from build123d import *

# Parameters (mm, degrees)
SKETCH1_W                 = 54.5
SKETCH1_H                 = 39
BOSS_EXTRUDE1_DEPTH       = 3
SKETCH10_R                = 7
CUT_EXTRUDE1_DEPTH        = 5
M2_CLEARANCE_HOLE1_D      = 2.4
M2_CLEARANCE_HOLE1_DEPTH  = 17
M2_CLEARANCE_HOLE1_TIP    = 0.721032743
SKETCH12_W                = 20
SKETCH12_H                = 5
BOSS_EXTRUDE2_DEPTH       = 20
SKETCH13_R                = 4.25
CUT_EXTRUDE2_DEPTH        = 5
SKETCH16_W                = 54.5
SKETCH16_H                = 5
BOSS_EXTRUDE4_DEPTH       = 12
F_8_CLEARANCE_HOLE1_D     = 4.4958
F_8_CLEARANCE_HOLE1_DEPTH = 17
F_8_CLEARANCE_HOLE1_TIP   = 1.350674586
RIB2_REACH                = 67.289
SKETCH20_WALL_W           = 150.605379482
SKETCH20_WALL_H           = 5
RIB4_REACH                = 67.289
SKETCH21_WALL_W           = 150.605379482
SKETCH21_WALL_H           = 5


with BuildPart() as part:
    # Sketch1 → Boss-Extrude1 (new body)
    with BuildSketch(Plane(origin=(0, 0, 0), x_dir=(1, 0, 0), z_dir=(0, 1, 0))):
        with Locations((-13.399543841, 8.129312584)):
            Rectangle(SKETCH1_W, SKETCH1_H)
    extrude(amount=BOSS_EXTRUDE1_DEPTH)

    # Sketch10 → Cut-Extrude1 (cut)
    with BuildSketch(Plane(origin=(0, 3, 0), x_dir=(1, 0, 0), z_dir=(0, 1, 0))):
        with Locations(Location((-13.399543841, 8.129312584, 0), (0, 0, 270))):
            Circle(SKETCH10_R)
    extrude(amount=-CUT_EXTRUDE1_DEPTH, mode=Mode.SUBTRACT)

    # M2 Clearance Hole1
    with Locations(Plane(origin=(-13.399543841, 3, -0.129312584), x_dir=(0, 0, 1), z_dir=(0, 1, 0))):
        with Locations((0, 0), (-8, 7.99475453), (-8, -7.99475453), (-16, 0)):
            Hole(M2_CLEARANCE_HOLE1_D / 2, depth=M2_CLEARANCE_HOLE1_DEPTH)
            with Locations((0, 0, -(M2_CLEARANCE_HOLE1_DEPTH + M2_CLEARANCE_HOLE1_TIP / 2))):  # 118° drill point
                Cone(0, M2_CLEARANCE_HOLE1_D / 2, M2_CLEARANCE_HOLE1_TIP, mode=Mode.SUBTRACT)

    # Sketch12 → Boss-Extrude2 (add)
    with BuildSketch(Plane(origin=(0, 3, 0), x_dir=(1, 0, 0), z_dir=(0, 1, 0))):
        with Locations((3.850456159, -8.870687416)):
            Rectangle(SKETCH12_W, SKETCH12_H)
        with Locations((-30.649543841, -8.870687416)):
            Rectangle(SKETCH12_W, SKETCH12_H)
    extrude(amount=BOSS_EXTRUDE2_DEPTH)

    # Sketch13 → Cut-Extrude2 (cut)
    with BuildSketch(Plane(origin=(0, 0, 6.370687416), x_dir=(-1, 0, 0), z_dir=(0, 0, -1))):
        with Locations((-3.850456159, 18)):
            Circle(SKETCH13_R)
        with Locations((30.649543841, 18)):
            Circle(SKETCH13_R)
    extrude(amount=-CUT_EXTRUDE2_DEPTH, mode=Mode.SUBTRACT)

    # Sketch16 → Boss-Extrude4 (add)
    with BuildSketch(Plane.XZ):
        with Locations((-13.399543841, 8.870687416)):
            Rectangle(SKETCH16_W, SKETCH16_H)
    extrude(amount=BOSS_EXTRUDE4_DEPTH)

    # #8 Clearance Hole1
    with Locations(Plane(origin=(-30.649543841, -8.2, 11.370687416), x_dir=(1, 0, 0), z_dir=(0, 0, 1))):
        with Locations((0, 0), (17.25, 0), (34.5, 0)):
            Hole(F_8_CLEARANCE_HOLE1_D / 2, depth=F_8_CLEARANCE_HOLE1_DEPTH)
            with Locations((0, 0, -(F_8_CLEARANCE_HOLE1_DEPTH + F_8_CLEARANCE_HOLE1_TIP / 2))):  # 118° drill point
                Cone(0, F_8_CLEARANCE_HOLE1_D / 2, F_8_CLEARANCE_HOLE1_TIP, mode=Mode.SUBTRACT)

    # Sketch20 wall → Rib2 (add, up to next)
    with BuildSketch(Plane(origin=(13.850456159, 10.5, 1.370687416), x_dir=(0, -0.832050294338, -0.554700196225), z_dir=(0, 0.554700196225, -0.832050294338)), mode=Mode.PRIVATE) as rib2_sk1:
        with Locations((0, 2.5)):
            Rectangle(SKETCH20_WALL_W, SKETCH20_WALL_H)
    rib2_tool1 = extrude(rib2_sk1.sketch, amount=-RIB2_REACH, mode=Mode.PRIVATE) - part.part
    add(rib2_tool1.solids().sort_by_distance((13.850456159, 10.5, 1.370687416))[0])

    # Sketch21 wall → Rib4 (add, up to next)
    with BuildSketch(Plane(origin=(-40.649543841, 10.5, 1.370687416), x_dir=(0, -0.832050294338, -0.554700196225), z_dir=(0, -0.554700196225, 0.832050294338)), mode=Mode.PRIVATE) as rib4_sk1:
        with Locations((0, 2.5)):
            Rectangle(SKETCH21_WALL_W, SKETCH21_WALL_H)
    rib4_tool1 = extrude(rib4_sk1.sketch, amount=RIB4_REACH, mode=Mode.PRIVATE) - part.part
    add(rib4_tool1.solids().sort_by_distance((-40.649543841, 10.5, 1.370687416))[0])


solid = part.part
Geometry: final body of the model. Coordinates: model frame, mm. A direction names the side the tool comes from. Coordinates: 2 decimals unless noted, no trailing zeros. Loops run counter-clockwise (first coordinate to the right, second up) from the corner with the lowest first, then second, coordinate; pieces in that order, holes last. Notation, with made-up numbers: (-37, 27.5) - (15, 27.5) arc R26 cw to (15, 65.5) - close; hole circle Ø5 at (-33.5, -26). An arc over 180 degrees is marked (long way). Put each result on its own line as item: value. Start each with the question number.
Q1. Cut plane D-D, the plane z = -10. Return loops of the section in (x, y).
Q2. Line query: line 1 (X direction, y = 2, z = 0); line 2 (X direction, y = 4, z = 9); line 3 (Y direction, x = 2, z = 8.5). Output: solid intervals per line, ascending.
Q3. Pull-direction query (Y, two-part tool) for faces 6 (the cylindrical face through (1.89, 14.23, 8.84)), 7 (the flat face through (-20, 0, -15)), 8 (the cylindrical face through (-4.206, 1.479, -8.173)), 9 (the flat face through (-38.115, 10.605, 1.441)); classes: released by +Y, released by -Y, zero draft, split by the parting line, or undercut.
Q4. Cut plane A-A, the plane y = -8.2. Return loops of the section in (x, z), and give its area (3 significant figures).
Q5. Cut plane B-B, the plane x = -25. Return loops of the section in (y, z), and give its area (3 significant figures).
Q6. Pin query (flat end, axial travel): pin 1 Ø10 at (x, z) = (3.5, -8.5) entering from +Y; pin 2 Ø5 at (x, y) = (-30.65, 18) entering from +Z; pin 3 Ø4 at (x, z) = (-2.5, -15) entering from -Y; pin 4 Ø13 at (x, y) = (-9, -7) entering from -Z. Return the tip coordinate at first contact, or that it passes through.
Q7. Cut plane C-C, the plane y = 7. Return loops of the section in (x, z).
Q8. Set-up query: faces 1 (the flat face through (8.85, 8, 2)), 2 (the cylindrical face through (-8.4, 1.52, -13.03)), 3 (the flat face through (-14, -5, 6.371)), 4 (the flat face through (-40.65, 5, 2)), 5 (the flat face through (-6.15, 13, 9)). Return all of +Z, -Z, +X, -X, +Y, -Y with unobstructed straight access to the full face (end or side cutting, diameter ignored); none if empty.
Filled sheet:
1. outline: (-40.65, 0) - (-20.14, 0) - (-20.14, 3) - (-40.65, 3) - close; (-6.65, 0) - (13.85, 0) - (13.85, 3) - (-6.65, 3) - close
2. line 1: -40.65 to -14.59, -12.21 to 13.85
2. line 2: -40.65 to -20.65, -6.15 to 13.85
2. line 3: -12 to -9.48, -6.92 to 14.17, 21.83 to 23
3. face 6: undercut
3. face 7: released by -Y
3. face 8: zero draft
3. face 9: released by +Y
4. outline: (-40.65, 6.37) - (-32.9, 6.37) - (-32.9, 11.37) - (-40.65, 11.37) - close; (-28.4, 6.37) - (-15.65, 6.37) - (-15.65, 11.37) - (-28.4, 11.37) - close; (-11.15, 6.37) - (1.6, 6.37) - (1.6, 11.37) - (-11.15, 11.37) - close; (6.1, 6.37) - (13.85, 6.37) - (13.85, 11.37) - (6.1, 11.37) - close
4. area: 205 mm²
5. outline: (-12, 6.37) - (0, 6.37) - (0, -27.63) - (3, -27.63) - (3, 6.37) - (23, 6.37) - (23, 11.37) - (-12, 11.37) - close
5. area: 277 mm²
6. pin 1: y = 3
6. pin 2: through
6. pin 3: y = 0
6. pin 4: z = 6.37
7. outline: (-40.65, -0.96) - (-35.65, -0.96) - (-35.65, 6.37) - (-20.65, 6.37) - (-20.65, 11.37) - (-40.65, 11.37) - close; (-6.15, 6.37) - (8.85, 6.37) - (8.85, -0.96) - (13.85, -0.96) - (13.85, 11.37) - (-6.15, 11.37) - close
8. face 1: -Z, +Y
8. face 2: +Y, -Y
8. face 3: -Z, +X, -X, -Y
8. face 4: +Z, -Z, -X, +Y, -Y
8. face 5: +Z, -Z, +Y
